Drawing for the job (mm, zero at the part's lowest x, y, z). Coordinates: 2 decimals unless noted, no trailing zeros. Write each loop counter-clockwise with the first axis right and the second up, starting at its lowest first coordinate (ties: lowest second). Pieces come first, ordered by that corner, then holes. Notation, with made-up numbers: (-21, 51.25) -> (37, 51.25) arc R17 cw to (37, 80.25) -> close; hole circle Ø11 at (-18.75, 9.25). An arc over 180 degrees is marked (long way). Answer as CSV lines item,"result".
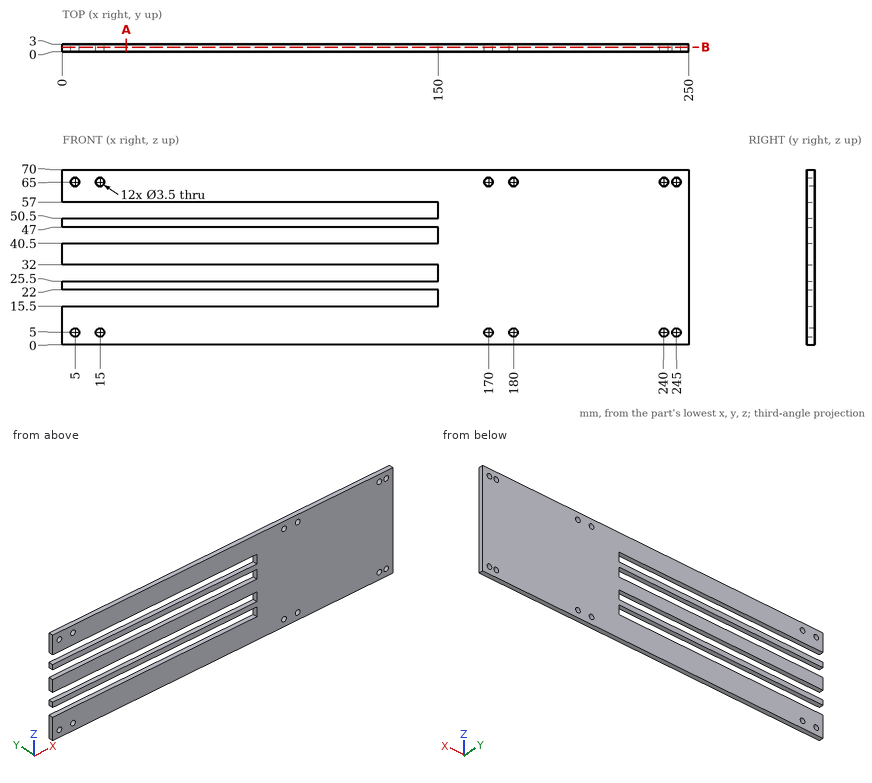
Item 1: Saw through at B-B on y = 1.8. State how many separate pieces and enclosed holes the cut face has, and give its area (3 significant figures).
Answer below:
separate pieces,"1"
enclosed holes,"12"
area,"13,500 mm2"
Item 2: Saw through at A-A on x = 25.5. Give the cut face in (y, z), and give its area (3 significant figures).
Answer below:
outline,"(0, 0) -> (3, 0) -> (3, 15.5) -> (0, 15.5) -> close; (0, 22) -> (3, 22) -> (3, 25.5) -> (0, 25.5) -> close; (0, 32) -> (3, 32) -> (3, 40.5) -> (0, 40.5) -> close; (0, 47) -> (3, 47) -> (3, 50.5) -> (0, 50.5) -> close; (0, 57) -> (3, 57) -> (3, 70) -> (0, 70) -> close"
area,"132 mm2"
Item 3: Wall check: line 1 (Z direction, x = 147, y = 1); line 2 (Z direction, x = 180, y = 1.45); line 3 (X direction, y = 1.85, z = 31). Give the ranges that are in metal, low to high. Write a range as from..to.
Answer below:
line 1,"z = 0..15.5, 22..25.5, 32..40.5, 47..50.5, 57..70"
line 2,"z = 0..3.25, 6.75..63.25, 66.75..70"
line 3,"x = 150..250"
Item 4: Flat gauge pin, fed straight in: pin 1 (0.9 mm diameter, centred on y = 2, z = 55.5, fed in from -X). Where does the tip first touch, or does it go through?
Answer below:
pin 1,"stops at x = 150"
